Answer from the drawing. Dimensions are ordinates in mm from the lowest x, y and z of the part. A direction names the side the tool comes from. Coordinates: 2 decimals unless noted, no trailing zeros. Order: outer loops, then holes, each group sorted by start corner. A loop starts at its lowest first (then second) coordinate and runs counter-clockwise, first axis right, second up. Notation, with made-up numbers: (-31, 35.25) -> (-16, 35.25) arc R29 cw to (-16, 59.25) -> close; hole circle Ø8 at (-33.75, 74.25). An arc over 180 degrees is marked (long way). Answer as a JSON object with one key per item and string values. Group by question number.
1) Consider L1, parallel to Y at x = 20, z = 3.25; L2, parallel to X at y = 80, z = 9. Determine where each line is inside the solid, lowest interval first.
2) A tool of negligible diameter and unlimited length cuts with its end or side. For the marked faces 5, 6, 7, 8 and 9, from which of +Z, -Z, +X, -X, +Y, -Y can it reach the whole face along a straight path? Write none if from no direction.
3) Given pin 1 (2 mm diameter, centred on y = 63, z = 5.5, fed in from +X); pin 2 (8 mm diameter, centred on x = 13.5, z = 20, fed in from +Y); pin 3 (5 mm diameter, centred on x = 62, z = 34, fed in from -Y), each flat-ended and moving along its own axis, determine where each tip first touches the part or whether it passes through.
4) Section A-A on z = 17 is taken. Determine the outline of the cut face in (x, y), and give its area (3 significant figures).
5) Section D-D on z = 8.5 is taken. Determine the outline of the cut face in (x, y).
6) Determine the mould class of the marked faces 1, 2, 3 and 4 for opening direction Y: released by +Y, released by -Y, zero draft, split by the parting line, or undercut.
7) Section C-C on x = 57.5 is taken. Determine the outline of the cut face in (y, z).
8) Section B-B on y = 24 is taken. Determine the outline of the cut face in (x, z), and give its area (3 significant figures).
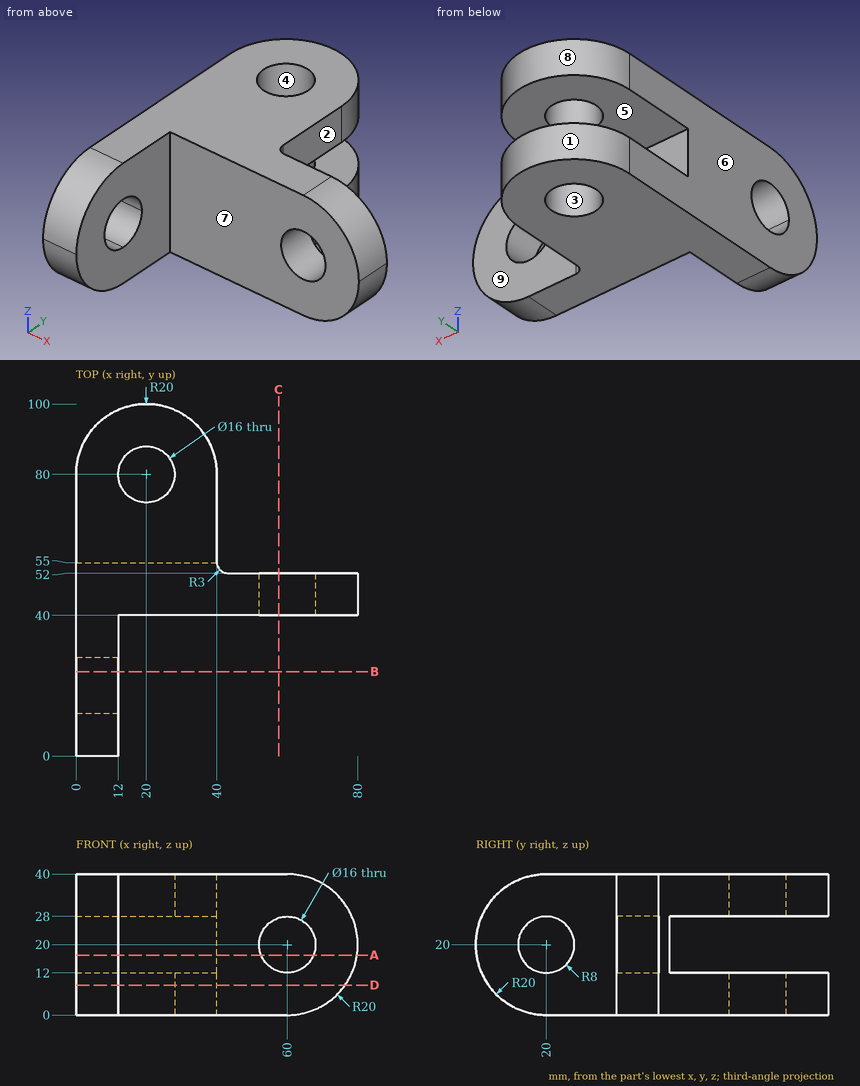
Worked answers:
{
 "1": {"L1": "y = 40 to 72, 88 to 100", "L2": "x = 0 to 12, 28 to 40"},
 "2": {"face 5": "+X, -X, +Y", "face 6": "+Z, -Z, -X, +Y, -Y", "face 7": "+Z, -Z, +X, -Y", "face 8": "+Z, -Z, +Y", "face 9": "+Z, -Z, +X, +Y"},
 "3": {"pin 1": "stops at x = 40", "pin 2": "stops at y = 55", "pin 3": "stops at y = 40"},
 "4": {"outline": "(0, 0.23) -> (12, 0.23) -> (12, 12.58) -> (0, 12.58) -> close; (0, 27.42) -> (12, 27.42) -> (12, 40) -> (52.58, 40) -> (52.58, 52) -> (43, 52) arc R3 cw to (40, 55) -> (0, 55) -> close; (67.42, 40) -> (79.77, 40) -> (79.77, 52) -> (67.42, 52) -> close", "area": "1,200 mm²"},
 "5": {"outline": "(0, 3.64) -> (12, 3.64) -> (12, 40) -> (76.36, 40) -> (76.36, 52) -> (43, 52) arc R3 cw to (40, 55) -> (40, 80) arc R20 ccw to (0, 80) -> close; hole circle Ø16 at (20, 80)"},
 "6": {"face 1": "released by +Y", "face 2": "zero draft", "face 3": "undercut", "face 4": "undercut"},
 "7": {"outline": "(40, 0) -> (52, 0) -> (52, 12.4) -> (40, 12.4) -> close; (40, 27.6) -> (52, 27.6) -> (52, 40) -> (40, 40) -> close"},
 "8": {"outline": "(0, 0) -> (12, 0) -> (12, 13.07) -> (0, 13.07) -> close; (0, 26.93) -> (12, 26.93) -> (12, 40) -> (0, 40) -> close", "area": "314 mm²"}
}
